Source: CAD feature listing. Evaluate the final solid. Frame: model axes, mm. Face numbers are marked on the shaded views. Give positions to 0.01 mm unless a question says otherwise; leave off trailing zeros. Write each loop counter-clockwise with the first axis right and the second up, starting at its lowest first coordinate (ties: lowest second). Pieces come first, ordered by that corner, then holes. Notation, with made-up numbers: M -26.5,41 L 28.5,41 A20 ccw 28.5,63 Z; hole C 30,7 d2. An arc over 180 degrees is marked long. Use CSV: the item, a comma, the result in double quotes. Start each with the question number.
from build123d import *

# Parameters (mm, degrees)
SKICA1_W                  = 75
SKICA1_H                  = 45
P_IDAT_VYSUNUT_M1_DEPTH   = 13
SKICA2_W                  = 71
SKICA2_H                  = 41
ODEBRAT_VYSUNUT_M1_DEPTH  = 12
ZAOBLIT1_R                = 2
ZKOSEN_2_SIZE             = 0.5
SKICA4_W                  = 8.5
SKICA4_H                  = 8.5
P_IDAT_VYSUNUT_M2_DEPTH   = 4.22
ZAOBLIT2_R                = 1
SKICA6_W                  = 92.209043038
SKICA6_H                  = 16.914138174
ODEBRAT_VYSUNUT_M3_DEPTH  = 64.22
SKICA5_W                  = 10.08575576
SKICA5_H                  = 9.3
ODEBRAT_VYSUNUT_M4_DEPTH  = 10.5
SKICA7_W                  = 4
SKICA7_H                  = 7.545536299
ODEBRAT_VYSUNUT_M5_DEPTH  = 1.9
SKICA8_W                  = 14.8
SKICA8_H                  = 7.292326558
ODEBRAT_VYSUNUT_M6_DEPTH  = 1.4
SKICA9_R                  = 1.45
ODEBRAT_VYSUNUT_M7_DEPTH  = 5
SKICA10_R                 = 2.2
SKICA10_R_2               = 1.75
P_IDAT_VYSUNUT_M3_DEPTH   = 1.5
ODEBRAT_START             = -2
SKICA11_R                 = 2.925
SKICA11_R_2               = 1.45
ODEBRAT_VYSUNUT_M8_DEPTH  = 2
SKICA12_R                 = 1
P_IDAT_VYSUNUT_M4_DEPTH   = 3
ODEBRAT_VYSUNUT_M14_DEPTH = 1
ZKOSEN_3_SIZE             = 2
ZKOSEN_4_SIZE             = 2


with BuildPart() as part:
    # Skica1 → Přidat vysunutím1 (new body)
    with BuildSketch(Plane.XY):
        Rectangle(SKICA1_W, SKICA1_H)
    extrude(amount=P_IDAT_VYSUNUT_M1_DEPTH)

    # Skica2 → Odebrat vysunutím1 (cut)
    with BuildSketch(Plane.XY.offset(13)):
        Rectangle(SKICA2_W, SKICA2_H)
    extrude(amount=-ODEBRAT_VYSUNUT_M1_DEPTH, mode=Mode.SUBTRACT)

    # Zaoblit1
    zaoblit1_edges = [part.edges().sort_by_distance(p)[0] for p in [
        (35.5, 20.5, 7),
        (35.5, -20.5, 7),
        (-35.5, -20.5, 7),
        (-35.5, 20.5, 7),
        (37.5, -22.5, 6.5),
        (-37.5, -22.5, 6.5),
        (-37.5, 22.5, 6.5),
        (37.5, 22.5, 6.5),
    ]]
    fillet(zaoblit1_edges, radius=ZAOBLIT1_R)

    # Zkosení2
    zkosen_2_edges = [part.edges().sort_by_distance(p)[0] for p in [
        (0, 22.5, 0),
        (37.5, 0, 0),
        (0, -22.5, 0),
        (-37.5, 0, 0),
        (-36.914213562, 21.914213562, 0),
        (-36.914213562, -21.914213562, 0),
        (36.914213562, -21.914213562, 0),
        (36.914213562, 21.914213562, 0),
    ]]
    chamfer(zkosen_2_edges, length=ZKOSEN_2_SIZE)

    # Skica4 → Přidat vysunutím2 (add)
    with BuildSketch(Plane.XY.offset(1)):
        with Locations((-32.664213562, 17.664213562)):
            Rectangle(SKICA4_W, SKICA4_H)
        with Locations((-32.664213562, -17.664213562)):
            Rectangle(SKICA4_W, SKICA4_H)
        with Locations((32.664213562, -17.664213562)):
            Rectangle(SKICA4_W, SKICA4_H)
        with Locations((32.664213562, 17.664213562)):
            Rectangle(SKICA4_W, SKICA4_H)
    extrude(amount=P_IDAT_VYSUNUT_M2_DEPTH)

    # Zaoblit2
    zaoblit2_edges = [part.edges().sort_by_distance(p)[0] for p in [
        (-28.414213562, 13.414213562, 3.11),
        (-28.414213562, -13.414213562, 3.11),
        (28.414213562, -13.414213562, 3.11),
        (28.414213562, 13.414213562, 3.11),
    ]]
    fillet(zaoblit2_edges, radius=ZAOBLIT2_R)

    # Skica6 → Odebrat vysunutím3 (cut)
    with BuildSketch(Plane.XZ.offset(22.5)):
        with Locations((-2.449143373, 13.457069087)):
            Rectangle(SKICA6_W, SKICA6_H)
    extrude(amount=-ODEBRAT_VYSUNUT_M3_DEPTH, mode=Mode.SUBTRACT)

    # Skica5 → Odebrat vysunutím4 (cut)
    with BuildSketch(Plane.XY.offset(13)):
        with Locations((-37.618064514, 2.55)):
            Rectangle(SKICA5_W, SKICA5_H)
    extrude(amount=-ODEBRAT_VYSUNUT_M4_DEPTH, mode=Mode.SUBTRACT)

    # Skica7 → Odebrat vysunutím5 (cut)
    with BuildSketch(Plane.XY.offset(5)):
        with Locations((14.5, 17.977231851)):
            Rectangle(SKICA7_W, SKICA7_H)
    extrude(amount=-ODEBRAT_VYSUNUT_M5_DEPTH, mode=Mode.SUBTRACT)

    # Skica8 → Odebrat vysunutím6 (cut)
    with BuildSketch(Plane.XY.offset(5)):
        with Locations((-0.1, 20.570563513)):
            Rectangle(SKICA8_W, SKICA8_H)
    extrude(amount=-ODEBRAT_VYSUNUT_M6_DEPTH, mode=Mode.SUBTRACT)

    # Skica9 → Odebrat vysunutím7 (cut, symmetric)
    with BuildSketch(Plane.XY.offset(1)):
        with Locations(Location((-32.114213562, 16.914213562, 0), (0, 0, 180))):
            Circle(SKICA9_R)
        with Locations(Location((-32.114213562, -16.914213562, 0), (0, 0, 180))):
            Circle(SKICA9_R)
        with Locations(Location((31.914213562, -16.914213562, 0), (0, 0, 180))):
            Circle(SKICA9_R)
        with Locations(Location((31.914213562, 16.914213562, 0), (0, 0, 180))):
            Circle(SKICA9_R)
    extrude(amount=ODEBRAT_VYSUNUT_M7_DEPTH, both=True, mode=Mode.SUBTRACT)

    # Skica10 → Přidat vysunutím3 (add)
    # profile 1 of 4: a face of its own
    with BuildSketch(Plane.XY.offset(5)):
        with Locations(Location((31.914213562, 16.914213562, 0), (0, 0, 180))):
            Circle(SKICA10_R)
        with Locations((31.914213562, 16.914213562)):
            Circle(SKICA10_R_2, mode=Mode.SUBTRACT)
    # profile 2 of 4: a face of its own
    with BuildSketch(Plane.XY.offset(5)):
        with Locations(Location((31.914213562, -16.914213562, 0), (0, 0, 180))):
            Circle(SKICA10_R)
        with Locations((31.914213562, -16.914213562)):
            Circle(SKICA10_R_2, mode=Mode.SUBTRACT)
    # profile 3 of 4: a face of its own
    with BuildSketch(Plane.XY.offset(5)):
        with Locations(Location((-32.114213562, -16.914213562, 0), (0, 0, 180))):
            Circle(SKICA10_R)
        with Locations((-32.114213562, -16.914213562)):
            Circle(SKICA10_R_2, mode=Mode.SUBTRACT)
    # profile 4 of 4: a face of its own
    with BuildSketch(Plane.XY.offset(5)):
        with Locations(Location((-32.114213562, 16.914213562, 0), (0, 0, 180))):
            Circle(SKICA10_R)
        with Locations((-32.114213562, 16.914213562)):
            Circle(SKICA10_R_2, mode=Mode.SUBTRACT)
    extrude(amount=P_IDAT_VYSUNUT_M3_DEPTH)

    # Skica11 → Odebrat vysunutím8 (cut)
    # profile 1 of 4: a face of its own
    with BuildSketch(Plane(origin=(0, 0, 0), x_dir=(-1, 0, 0), z_dir=(0, 0, -1)).offset(ODEBRAT_START)):
        with Locations((32.114213562, -16.914213562)):
            Circle(SKICA11_R)
        with Locations((32.114213562, -16.914213562)):
            Circle(SKICA11_R_2, mode=Mode.SUBTRACT)
    # profile 2 of 4: a face of its own
    with BuildSketch(Plane(origin=(0, 0, 0), x_dir=(-1, 0, 0), z_dir=(0, 0, -1)).offset(ODEBRAT_START)):
        with Locations((-31.914213562, -16.914213562)):
            Circle(SKICA11_R)
        with Locations((-31.914213562, -16.914213562)):
            Circle(SKICA11_R_2, mode=Mode.SUBTRACT)
    # profile 3 of 4: a face of its own
    with BuildSketch(Plane(origin=(0, 0, 0), x_dir=(-1, 0, 0), z_dir=(0, 0, -1)).offset(ODEBRAT_START)):
        with Locations((-31.914213562, 16.914213562)):
            Circle(SKICA11_R)
        with Locations((-31.914213562, 16.914213562)):
            Circle(SKICA11_R_2, mode=Mode.SUBTRACT)
    # profile 4 of 4: a face of its own
    with BuildSketch(Plane(origin=(0, 0, 0), x_dir=(-1, 0, 0), z_dir=(0, 0, -1)).offset(ODEBRAT_START)):
        with Locations((32.114213562, 16.914213562)):
            Circle(SKICA11_R)
        with Locations((32.114213562, 16.914213562)):
            Circle(SKICA11_R_2, mode=Mode.SUBTRACT)
    extrude(amount=ODEBRAT_VYSUNUT_M8_DEPTH, mode=Mode.SUBTRACT)

    # Skica12 → Přidat vysunutím4 (add)
    with BuildSketch(Plane.XY.offset(1)):
        with Locations(Location((23.314213562, -16.6, 0), (0, 0, 180))):
            Circle(SKICA12_R)
        with Locations(Location((19.664213562, -16.6, 0), (0, 0, 180))):
            Circle(SKICA12_R)
    extrude(amount=P_IDAT_VYSUNUT_M4_DEPTH)

    # Skica13 → Odebrat vysunutím14 (cut)
    with BuildSketch(Plane.XY.offset(1)):
        with BuildLine():
            ThreePointArc((24.814213562, -16.6), (23.314213562, -18.1), (21.814213562, -16.6))
            Line((21.814213562, -16.6), (21.814213562, -9.556250206))
            Line((21.814213562, -9.556250206), (21.514213562, -9.556250206))
            Line((21.514213562, -9.556250206), (21.464213562, -9.556250206))
            Line((21.464213562, -9.556250206), (21.164213562, -9.556250206))
            Line((21.164213562, -9.556250206), (21.164213562, -16.6))
            ThreePointArc((21.164213562, -16.6), (19.664213562, -18.1), (18.164213562, -16.6))
            Line((18.164213562, -16.6), (18.164213562, -9.556250206))
            Line((18.164213562, -9.556250206), (17.814213562, -9.556250206))
            Line((17.814213562, -9.556250206), (17.814213562, -16.6))
            ThreePointArc((17.814213562, -16.6), (19.512144499, -18.443739407), (21.489213562, -16.903108891))
            ThreePointArc((21.489213562, -16.903108891), (23.466282626, -18.443739407), (25.164213562, -16.6))
            Line((25.164213562, -16.6), (25.164213562, -9.556250206))
            Line((25.164213562, -9.556250206), (24.814213562, -9.556250206))
            Line((24.814213562, -9.556250206), (24.814213562, -16.6))
        make_face()
    extrude(amount=-ODEBRAT_VYSUNUT_M14_DEPTH, mode=Mode.SUBTRACT)

    # Zkosení3
    # the kernel refuses this chamfer: 2 mm, written as the material it takes off along each edge
    with BuildSketch(Plane(origin=(31.914213562, 16.914213562, 2), x_dir=(-1, 0, 0), z_dir=(0, -1, 0))) as zkosen_3_piece_1_section:
        Polygon((1.45 + ZKOSEN_3_SIZE, 0), (1.45, -ZKOSEN_3_SIZE), (1.45, 0), align=None)
    zkosen_3_piece_1 = revolve(axis=Axis((31.914213562, 16.914213562, 2), (0, 0, -1)), mode=Mode.PRIVATE)
    zkosen_3_piece_1 = zkosen_3_piece_1 & Plane(origin=(31.914213562, 16.914213562, 3.26993651), x_dir=(-1, 0, 0), z_dir=(0, 0, 1)) * Cylinder(2.925, 14, mode=Mode.PRIVATE)
    add(zkosen_3_piece_1, mode=Mode.SUBTRACT)
    with BuildSketch(Plane(origin=(-32.114213562, -16.914213562, 2), x_dir=(-1, 0, 0), z_dir=(0, -1, 0))) as zkosen_3_piece_2_section:
        Polygon((1.45 + ZKOSEN_3_SIZE, 0), (1.45, -ZKOSEN_3_SIZE), (1.45, 0), align=None)
    zkosen_3_piece_2 = revolve(axis=Axis((-32.114213562, -16.914213562, 2), (0, 0, -1)), mode=Mode.PRIVATE)
    zkosen_3_piece_2 = zkosen_3_piece_2 & Plane(origin=(-32.114213562, -16.914213562, 3.26993651), x_dir=(-1, 0, 0), z_dir=(0, 0, 1)) * Cylinder(2.925, 14, mode=Mode.PRIVATE)
    add(zkosen_3_piece_2, mode=Mode.SUBTRACT)

    # Zkosení4
    # the kernel refuses this chamfer: 2 mm, written as the material it takes off along each edge
    with BuildSketch(Plane(origin=(31.914213562, -16.914213562, 2), x_dir=(-1, 0, 0), z_dir=(0, -1, 0))) as zkosen_4_piece_1_section:
        Polygon((1.45 + ZKOSEN_4_SIZE, 0), (1.45, -ZKOSEN_4_SIZE), (1.45, 0), align=None)
    zkosen_4_piece_1 = revolve(axis=Axis((31.914213562, -16.914213562, 2), (0, 0, -1)), mode=Mode.PRIVATE)
    zkosen_4_piece_1 = zkosen_4_piece_1 & Plane(origin=(31.914213562, -16.914213562, 3.26993651), x_dir=(-1, 0, 0), z_dir=(0, 0, 1)) * Cylinder(2.925, 14, mode=Mode.PRIVATE)
    add(zkosen_4_piece_1, mode=Mode.SUBTRACT)
    with BuildSketch(Plane(origin=(-32.114213562, 16.914213562, 2), x_dir=(-1, 0, 0), z_dir=(0, -1, 0))) as zkosen_4_piece_2_section:
        Polygon((1.45 + ZKOSEN_4_SIZE, 0), (1.45, -ZKOSEN_4_SIZE), (1.45, 0), align=None)
    zkosen_4_piece_2 = revolve(axis=Axis((-32.114213562, 16.914213562, 2), (0, 0, -1)), mode=Mode.PRIVATE)
    zkosen_4_piece_2 = zkosen_4_piece_2 & Plane(origin=(-32.114213562, 16.914213562, 3.26993651), x_dir=(-1, 0, 0), z_dir=(0, 0, 1)) * Cylinder(2.925, 14, mode=Mode.PRIVATE)
    add(zkosen_4_piece_2, mode=Mode.SUBTRACT)


solid = part.part
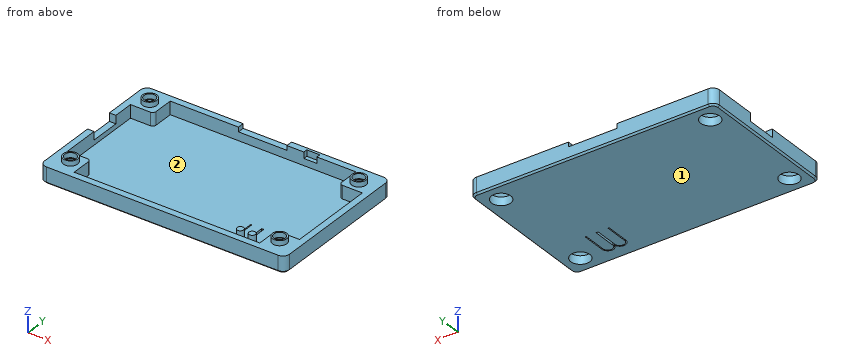
1. Section C-C on z = 5.75. Return loops of the section in (x, y), then the cut area to 3 significant figures.
2. Line query: probe 1 along Y at (x, z) = (23.5, 1.5); probe 2 along X at (y, z) = (16, 3.75); probe 3 along Y at (x, z) = (-13.5, 1.25). Output: solid intervals per line, ascending.
3. Section B-B on y = 4.5. Return loops of the section in (x, z), then the cut area to 4 significant figures.
4. Section A-A on x = -5. Return loops of the section in (y, z), then the cut area to 4 significant figures.
5. Pull-direction query (Y, two-part tool) for the marked faces 1 and 2; classes: released by +Y, released by -Y, zero draft, split by the parting line, or undercut.
6. First-contact query: pin 1 (3 mm diameter, centred on x = 17.5, y = -4.5, fed in from -Z); pin 2 (10 mm diameter, centred on x = 23, y = 1.5, fed in from +Z); pin 3 (0.6 mm diameter, centred on x = 19, y = -16.5, fed in from +Z); pin 4 (3.5 mm diameter, centred on x = -32.11, y = 16.91, fed in from -Z). Flat tips, straight axial feed; report the tip coordinate or a pass-through.
7. Section D-D on x = 13.5. Return loops of the section in (y, z).
Resolved:
1,outline,"C -32.11,-16.91 d4.4; C -32.11,16.91 d4.4; C 31.91,-16.91 d4.4; C 31.91,16.91 d4.4; hole C -32.11,-16.91 d3.5; hole C -32.11,16.91 d3.5; hole C 31.91,-16.91 d3.5; hole C 31.91,16.91 d3.5"
1,area,"22.3 mm2"
2,probe 1,"y = -22.5 to -20.5, -17.58 to -15.62, 20.5 to 22.5"
2,probe 2,"x = -37.5 to -33.55, -30.68 to -28.41, 28.41 to 30.48, 33.35 to 37.5"
2,probe 3,"y = -22.5 to -20.5, 20.5 to 22.5"
3,outline,"M -37.5,0.5 L -37,0 L 37,0 L 37.5,0.5 L 37.5,5 L 35.5,5 L 35.5,1 L -35.5,1 L -35.5,2.5 L -37.5,2.5 Z"
3,area,"85.75 mm2"
4,outline,"M -22.5,0.5 L -22,0 L 22,0 L 22.5,0.5 L 22.5,3.6 L 20.5,3.6 L 20.5,1 L -20.5,1 L -20.5,5 L -22.5,5 Z"
4,area,"57.95 mm2"
5,face 1,"zero draft"
5,face 2,"undercut"
6,pin 1,"stops at z = 0"
6,pin 2,"stops at z = 1"
6,pin 3,"stops at z = 4"
6,pin 4,"stops at z = 3.69"
7,outline,"M -22.5,0.5 L -22,0 L 22,0 L 22.5,0.5 L 22.5,5 L 21.75,5 L 21.75,3.1 L 20.5,3.1 L 20.5,1 L -20.5,1 L -20.5,5 L -22.5,5 Z"
